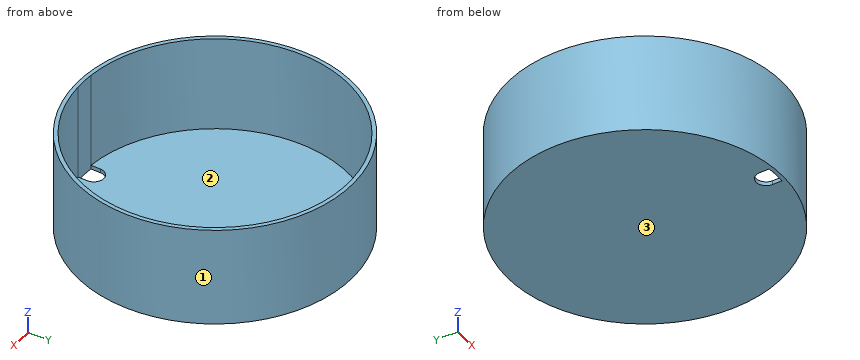
from build123d import *

# Parameters (mm, degrees)
F0_R     = 34.5
F1_DEPTH = 1
F2_DEPTH = 25


with BuildPart() as f1:
    # F0 (on Top) → F1 (new body)
    with BuildSketch(Plane.XY):
        Circle(F0_R)
        with BuildLine():
            ThreePointArc((-2.5, -33.406586), (-22.787058, 24.556058), (33.5, 0))
            ThreePointArc((33.5, 0), (24.556058, -22.787058), (2.5, -33.406586))
            ThreePointArc((2.5, -33.406586), (0, -33.5), (-2.5, -33.406586))
        make_face(mode=Mode.SUBTRACT)
        with BuildLine():
            ThreePointArc((2.5, -33.406586), (24.556058, -22.787058), (33.5, 0))
            ThreePointArc((33.5, 0), (-22.787058, 24.556058), (-2.5, -33.406586))
            Line((-2.5, -33.406586), (-2.5, -31))
            ThreePointArc((-2.5, -31), (0, -28.5), (2.5, -31))
            Line((2.5, -31), (2.5, -33.406586))
        make_face()
    extrude(amount=F1_DEPTH)

    # F0 (on Top) → F2 (join)
    with BuildSketch(Plane.XY):
        Circle(F0_R)
        with BuildLine():
            ThreePointArc((-2.5, -33.406586), (-22.787058, 24.556058), (33.5, 0))
            ThreePointArc((33.5, 0), (24.556058, -22.787058), (2.5, -33.406586))
            ThreePointArc((2.5, -33.406586), (0, -33.5), (-2.5, -33.406586))
        make_face(mode=Mode.SUBTRACT)
    extrude(amount=F2_DEPTH)


solid = f1.part
Read the model definition and answer for the solid it produces. Units are mm, in the model's axes. Face numbers are marked on the shaded views. Round coordinates to 2 decimals unless told otherwise and drop trailing zeros. Write each loop counter-clockwise with the first axis right and the second up, starting at its lowest first coordinate (ties: lowest second). Pieces come first, ordered by that corner, then holes. Notation, with made-up numbers: (-33.75, 57) - (-21.75, 57) arc R22 ccw to (-21.75, 73) - close; hole circle Ø2 at (66, 59). An arc over 180 degrees is marked (long way). One line per question, with ' | ' between items. Start each with the question number.
1. Find the intervals of material crossed by probe 1 along Y at (x, z) = (0, 14.5); probe 2 along Z at (x, y) = (-23, 16); probe 3 along X at (y, z) = (11.5, 4.5), in increasing order. Write a range as [from, to].
2. Section D-D (x = 10) is taken. Determine the outline of the cut face in (y, z).
3. Section A-A (x = 0) is taken. Determine the outline of the cut face in (y, z).
4. Each of these flat-tipped pins is pushed along its axis until it touches: pin 1 (6 mm diameter, centred on x = -1, z = 20.5, fed in from -Y); pin 2 (1.5 mm diameter, centred on x = 23, y = -16.5, fed in from +Z); pin 3 (10 mm diameter, centred on y = -22, z = 8.5, fed in from +X). Where does it stop, or does it pass through?
5. For a pull along Y with two mould halves and no side action, classify the marked faces 1, 2 and 3 as +Y half, -Y half, draft (parallel to the pull), parting line (faces both ways), or undercut.
6. Section C-C (y = -5) is taken. Determine the outline of the cut face in (x, z).
7. Section B-B (z = 19.5) is taken. Determine the outline of the cut face in (x, y), and give its area (3 significant figures).
Filled in:
1) probe 1: [-34.5, -33.5], [33.5, 34.5] | probe 2: [0, 1] | probe 3: [-32.53, -31.46], [31.46, 32.53]
2) outline: (-33.02, 0) - (33.02, 0) - (33.02, 25) - (31.97, 25) - (31.97, 1) - (-31.97, 1) - (-31.97, 25) - (-33.02, 25) - close
3) outline: (-34.5, 0) - (-33.5, 0) - (-33.5, 25) - (-34.5, 25) - close; (-28.5, 0) - (34.5, 0) - (34.5, 25) - (33.5, 25) - (33.5, 1) - (-28.5, 1) - close
4) pin 1: y = -34.5 | pin 2: z = 1 | pin 3: x = 30.02
5) face 1: parting line | face 2: undercut | face 3: draft
6) outline: (-34.14, 0) - (34.14, 0) - (34.14, 25) - (33.12, 25) - (33.12, 1) - (-33.12, 1) - (-33.12, 25) - (-34.14, 25) - close
7) outline: circle Ø69 at (0, 0); hole (-2.5, -33.41) arc R33.5 ccw to (2.5, -33.41) arc R33.5 ccw (long way) to start | area: 214 mm²
